Here's how the part is built. I have some questions about the finished solid (model axes, mm). A direction names the side the tool comes from. Give positions to 0.01 mm unless a question says otherwise; leave off trailing zeros. Loops run counter-clockwise (first coordinate to the right, second up) from the corner with the lowest first, then second, coordinate; pieces in that order, holes last.
Q1. I need wall thicknesses on probe 1 along Z at (x, y) = (-2, 0.2); probe 2 along Z at (x, y) = (-7.5, 1.6); probe 3 along X at (y, z) = (1.05, -15.5). Which ranges of each line are inside material? Lowest first, please.
Q2. Suppose I cut it at D-D (x = 12). List the corners of the cut face in (y, z) for me.
Q3. For faces 1 (the face through (-1.143, 2, 16)), 2 (the face through (11.392, 2, -10)), 3 (the face through (-8, 2, 24.689)), 4 (the face through (14, 2, 19.939)), 5 (the face through (-16.192, 2, 1)), which set-ups out of +Z, -Z, +X, -X, +Y, -Y let a thin tool reach every point of the face, with its end or its side?
Q4. Suppose I cut it at A-A (z = -5.5). List the corners of the cut face in (x, y) for me.
Q5. I'm going to push flat-ended pins straight in: P1, Ø1.2, axis at x = 2.5, y = 3, coming from the +Z side; P2, Ø2.5, axis at y = 1.5, z = 21.5, coming from the +X side. Where does each tip first touch, or does it pass through?
Q6. Suppose I cut it at C-C (y = 4). List the corners of the cut face in (x, z) for me, and give its area (3 significant figures).
Q7. Suppose I cut it at B-B (x = 7.5). List the corners of the cut face in (y, z) for me, and give its area (3 significant figures).
Q8. Thinking about a two-plate mould opening in X: for faces 6 (the face through (-13.121, 2.382, -10.867)), 7 (the face through (-10.922, 2, 22)), 8 (the face through (0, 2, -19.939)), which applies, pulls with the +X half, pulls with the -X half, needs draft (parallel to the pull), parting line crosses it, or undercut?
```python
from build123d import *

# Parameters (mm, degrees)
SKETCH1_W           = 32.385
SKETCH1_H           = 39.878
SKETCH1_W_2         = 22.7838
SKETCH1_H_2         = 12.3698
SKETCH1_W_3         = 5.842
SKETCH1_H_3         = 4.7498
BOSS_EXTRUDE1_DEPTH = 4.699
SKETCH2_W           = 1.143
SKETCH2_H           = 8.89
CUT_EXTRUDE1_DEPTH  = 30.896730635
FILLET1_R           = 1.27
SKETCH3_R           = 1.0795
CUT_EXTRUDE2_DEPTH  = 30.896730635


with BuildPart() as part:
    # Sketch1 → Boss-Extrude1 (new body)
    # profile 1 of 3: a face of its own
    with BuildSketch(Plane(origin=(0, 0, 0), x_dir=(1, 0, 0), z_dir=(0, 1, 0))):
        Rectangle(SKETCH1_W, SKETCH1_H)
        with Locations((0, 10.0711)):
            Rectangle(SKETCH1_W_2, SKETCH1_H_2, mode=Mode.SUBTRACT)
    # profile 2 of 3: a face of its own
    with BuildSketch(Plane(origin=(0, 0, 0), x_dir=(1, 0, 0), z_dir=(0, 1, 0))):
        with Locations((-8.001, -22.3139)):
            Rectangle(SKETCH1_W_3, SKETCH1_H_3)
    # profile 3 of 3: a face of its own
    with BuildSketch(Plane(origin=(0, 0, 0), x_dir=(1, 0, 0), z_dir=(0, 1, 0))):
        with Locations((8.001, -22.3139)):
            Rectangle(SKETCH1_W_3, SKETCH1_H_3)
    extrude(amount=BOSS_EXTRUDE1_DEPTH)

    # Sketch2 → Cut-Extrude1 (cut, through all)
    with BuildSketch(Plane(origin=(0, 4.699, 0), x_dir=(1, 0, 0), z_dir=(0, 1, 0))):
        Polygon((-2.0955, -11.049), (-1.143, -11.049), (0, -11.049), (1.143, -11.049), (2.0955, -11.049), (2.0955, -7.3914), (-2.0955, -7.3914), align=None)
        with Locations((0.5715, -15.494)):
            Rectangle(SKETCH2_W, SKETCH2_H)
        with Locations((-0.5715, -15.494)):
            Rectangle(SKETCH2_W, SKETCH2_H)
    extrude(amount=-CUT_EXTRUDE1_DEPTH, mode=Mode.SUBTRACT)

    # Fillet1
    fillet1_edges = [part.edges().sort_by_distance(p)[0] for p in [
        (16.1925, 2.3495, -19.939),
        (-16.1925, 2.3495, -19.939),
    ]]
    fillet(fillet1_edges, radius=FILLET1_R)

    # Sketch3 → Cut-Extrude2 (cut, through all)
    with BuildSketch(Plane(origin=(0, 4.699, 0), x_dir=(1, 0, 0), z_dir=(0, 1, 0))):
        with Locations(Location((13.85062, 10.0711, 0), (0, 0, 270))):
            Circle(SKETCH3_R)
        with Locations(Location((-13.85062, 10.0711, 0), (0, 0, 270))):
            Circle(SKETCH3_R)
    extrude(amount=-CUT_EXTRUDE2_DEPTH, mode=Mode.SUBTRACT)


solid = part.part
```
Solutions:
1. probe 1: z = -19.94 to -16.26, -3.89 to 7.39, 11.05 to 19.94
1. probe 2: z = -19.94 to -16.26, -3.89 to 24.69
1. probe 3: x = -16.19 to -11.39, 11.39 to 16.19
2. outline: (0, -19.94) - (4.7, -19.94) - (4.7, 19.94) - (0, 19.94) - close
3. face 1: +Z, +Y, -Y
3. face 2: +Y, -Y
3. face 3: +Z, +X, -X, +Y, -Y
3. face 4: +Z, +X, +Y, -Y
3. face 5: +Z, -Z, -X, +Y, -Y
4. outline: (-16.19, 0) - (-11.39, 0) - (-11.39, 4.7) - (-16.19, 4.7) - close; (11.39, 0) - (16.19, 0) - (16.19, 4.7) - (11.39, 4.7) - close
5. P1: stops at z = 19.94
5. P2: stops at x = 10.92
6. outline: (-16.19, -18.67) arc R1.27 ccw to (-14.92, -19.94) - (14.92, -19.94) arc R1.27 ccw to (16.19, -18.67) - (16.19, 19.94) - (10.92, 19.94) - (10.92, 24.69) - (5.08, 24.69) - (5.08, 19.94) - (1.14, 19.94) - (1.14, 11.05) - (2.1, 11.05) - (2.1, 7.39) - (-2.1, 7.39) - (-2.1, 11.05) - (-1.14, 11.05) - (-1.14, 19.94) - (-5.08, 19.94) - (-5.08, 24.69) - (-10.92, 24.69) - (-10.92, 19.94) - (-16.19, 19.94) - close; hole circle Ø2.16 at (-13.85, -10.07); hole (-11.39, -16.26) - (11.39, -16.26) - (11.39, -3.89) - (-11.39, -3.89) - close; hole circle Ø2.16 at (13.85, -10.07)
6. area: 1,020 mm2
7. outline: (0, -19.94) - (4.7, -19.94) - (4.7, -16.26) - (0, -16.26) - close; (0, -3.89) - (4.7, -3.89) - (4.7, 24.69) - (0, 24.69) - close
7. area: 152 mm2
8. face 6: undercut
8. face 7: pulls with the -X half
8. face 8: needs draft
